```python
from build123d import *

# Parameters (mm, degrees)
SKETCH1_R           = 5.25
SKETCH1_R_2         = 4.5
BOSS_EXTRUDE1_DEPTH = 5
CUT_EXTRUDE1_DEPTH  = 5
CUT_EXTRUDE2_DEPTH  = 2
SKETCH6_R           = 2
CUT_EXTRUDE4_DEPTH  = 0.35


with BuildPart() as part:
    # Sketch1 → Boss-Extrude1 (new body)
    with BuildSketch(Plane(origin=(0, 0, 0), x_dir=(1, 0, 0), z_dir=(0, 1, 0))):
        with Locations(Location((0, 0, 0), (0, 0, 270))):
            Circle(SKETCH1_R)
        with Locations(Location((0, 0, 0), (0, 0, 270))):
            Circle(SKETCH1_R_2, mode=Mode.SUBTRACT)
    extrude(amount=BOSS_EXTRUDE1_DEPTH)

    # Sketch2 → Cut-Extrude1 (cut)
    with BuildSketch(Plane(origin=(0, 0, 0), x_dir=(1, 0, 0), z_dir=(0, 1, 0))):
        Polygon((1.327689147, 3.795637322), (1.327689147, 5.701107087), (-1.5, 5.701107087), (-1.5, 3.701107087), align=None)
    extrude(amount=CUT_EXTRUDE1_DEPTH, mode=Mode.SUBTRACT)

    # Sketch4 → Revolve1 (revolve)
    with BuildSketch(Plane.XY):
        with BuildLine():
            Line((5.25, 5), (0, 5))
            Line((0, 5), (0, 10.18))
            ThreePointArc((0, 10.18), (3.687644912, 8.667004979), (5.25, 5))
        make_face()
    revolve(axis=Axis((0, 5, 0), (0, 1, 0)))

    # Sketch5 → Cut-Extrude2 (cut)
    with BuildSketch(Plane(origin=(0, 5, 0), x_dir=(-1, 0, 0), z_dir=(0, -1, 0))):
        with BuildLine():
            Line((1.5, 3.436931771), (1.5, 6))
            Line((1.5, 6), (-1.327689147, 6))
            Line((-1.327689147, 6), (-1.327689147, 3.507098734))
            ThreePointArc((-1.327689147, 3.507098734), (-0.093024772, -3.748846008), (1.5, 3.436931771))
        make_face()
    extrude(amount=-CUT_EXTRUDE2_DEPTH, mode=Mode.SUBTRACT)

    # Sketch6 → Cut-Extrude4 (cut)
    with BuildSketch(Plane(origin=(0, 10.29, 0), x_dir=(-1, 0, 0), z_dir=(0, -1, 0))):
        Circle(SKETCH6_R)
    extrude(amount=CUT_EXTRUDE4_DEPTH, mode=Mode.SUBTRACT)

    # Sweep1: sweep along a path in Sketch9
    with BuildLine(Plane(origin=(0, 1.5, 0), x_dir=(-1, 0, 0), z_dir=(0, -1, 0))) as sweep1_path:
        ThreePointArc((1.5, 4.242640687), (-0.090752997, -4.499084784), (-1.327689147, 4.299679236))
    # Friction Bump → Sweep1 (sweep)
    with BuildSketch(Plane.ZY.offset(-1.327689147)):
        Polygon((-4.299679236, 2.026185405), (-4.299679236, 1.426185405), (-4.099679236, 1.658472971), (-4.099679236, 1.7942723), align=None)
    sweep(path=sweep1_path.line)


solid = part.part
```
Read the model definition and answer for the solid it produces. Units are mm, in the model's axes. A direction names the side the tool comes from. Give positions to 0.01 mm unless a question says otherwise; leave off trailing zeros. Write each loop counter-clockwise with the first axis right and the second up, starting at its lowest first coordinate (ties: lowest second). Pieces come first, ordered by that corner, then holes. Notation, with made-up numbers: M -32,54 L -15,54 A34 ccw -15,89 Z; hole C 56.5,-0.5 d8. An arc over 180 degrees is marked long. Put each result on its own line as item: value. Start each with the question number.
1. The part is cut by section C-C, the plane y = 5.25. Give the vertices of the cut face in (x, z), and give its area (3 significant figures).
2. Which of the six approach directions +Z, -Z, +X, -X, +Y, -Y give full straight-line access (tool end or side, diameter ignored) to faces 1 (the flat face through (1, 5, 4)), 2 (the flat face through (-1.5, 4.2, -4.4)), 3 (the cylindrical face through (0.238, 5.986, 3.742)), 4 (the flat face through (1.328, 4.2, -4.5)), 5 (the flat face through (0, 0, 5))?
3. Each of these flat-tipped pins is pushed along its axis until it touches: pin 1 Ø0.5 at (y, z) = (3, -4) entering from +X; pin 2 Ø1 at (y, z) = (2.5, 2.5) entering from +X; pin 3 Ø4.5 at (x, z) = (-0.5, -0.5) entering from -Y. Where does it stop, or does it pass through?
4. For a pull along Z with two mould halves and no side action, classify faces 6 (the flat face through (0, 9.94, 0)), 7 (the cylindrical face through (-0.12, 2.46, 5.25)), 8 (the cylindrical face through (-0.1, 3.5, 4.5)) as released by +Z, released by -Z, zero draft, split by the parting line, or undercut.
5. The part is cut by section A-A, the plane y = 4. Give the vertices of the cut face in (x, z).
6. Consider line 1 along X through (y, z) = (2.8, 0); line 2 along Y through (x, z) = (0.75, -1.25); line 3 along X through (y, z) = (5.75, 3). Determine where each line is inside the solid, lowest interval first.
7. The part is cut by section B-B, the plane y = 9.25. Give the vertices of the cut face in (x, z).
Final values:
1. outline: M -1.5,-5.02 L -1.5,-3.44 A3.75 cw long 1.33,-3.51 L 1.33,-5.07 A5.24 ccw long Z
1. area: 37.8 mm²
2. face 1: none
2. face 2: -Z
2. face 3: -Y
2. face 4: -Z, -Y
2. face 5: +Z, -Z, +X, -X, -Y
3. pin 1: stops at x = 3.67
3. pin 2: stops at x = 4.85
3. pin 3: stops at y = 7
4. face 6: zero draft
4. face 7: split by the parting line
4. face 8: undercut
5. outline: M -1.5,-5.03 L -1.5,-4.24 A4.5 cw long 1.33,-4.3 L 1.33,-5.08 A5.25 ccw long Z
6. line 1: x = -5.25 to -4.5, 4.5 to 5.25
6. line 2: y = 7 to 9.94
6. line 3: x = -4.23 to -2.25, 2.25 to 4.23
7. outline: C 0,0 d5.97
